Autodesk Inventor part; units mm, degrees
ref_plane "YZ Plane" through (0, 0, 0) normal (1, 0, 0) x (0, 1, 0)
ref_plane "XZ Plane" through (0, 0, 0) normal (0, 1, 0) x (-1, 0, 0)
ref_plane "XY Plane" through (0, 0, 0) normal (0, 0, 1) x (1, 0, 0)
sketch "Sketch1" plane through (0, 0, 0) normal (0, 1, 0) x (-1, 0, 0)
  circle A0 centre (0, 0) radius 6.35
  circle A1 centre (0, 0) radius 3.175
  line L0 (0, 0) -> (-25.4, 0)
  line L1 (0, 0) -> (12.7, -21.997)
  line L2 (0, 0) -> (12.7, 21.997)
  line L3 (12.0126, 22.3939) -> (13.3874, 21.6002)
  line L4 (13.3874, 21.6002) -> (-0.6874, 0.3969) construction
  line L5 (0.6874, -0.3969) -> (12.0126, 22.3939) construction
  line L6 (0, -0.7937) -> (0, 0)
  line L7 (0, 0.7937) -> (-25.4, -0.7937) construction
  line L8 (-25.4, 0.7937) -> (0, -0.7937) construction
  line L9 (0.6874, 0.3969) -> (12.0126, -22.3939) construction
  line L10 (13.3874, -21.6002) -> (-0.6874, -0.3969) construction
  line L11 (-25.4, -0.7937) -> (-3.0742, -0.7937)
  line L12 (-3.0742, 0.7937) -> (-25.4, 0.7937)
  line L13 (0.8497, 3.0592) -> (12.0126, 22.3939)
  line L14 (13.3874, 21.6002) -> (2.2245, 2.2654)
  line L15 (2.2245, -2.2654) -> (13.3874, -21.6002)
  line L16 (12.0126, -22.3939) -> (0.8497, -3.0592)
  line L17 (-25.4, 0) -> (-50.8, 0)
  line L18 (12.7, -21.997) -> (25.4, -43.9941)
  line L19 (12.7, 21.997) -> (25.4, 43.9941)
  line L20 (26.0874, 43.5972) -> (13.3874, 21.6002)
  line L21 (13.3874, 21.6002) -> (12.0126, 22.3939)
  line L22 (12.0126, 22.3939) -> (24.7126, 44.391)
  line L23 (24.7126, 44.391) -> (26.0874, 43.5972)
  line L24 (26.0874, 43.5972) -> (12.0126, 22.3939) construction
  line L25 (13.3874, 21.6002) -> (24.7126, 44.391) construction
  line L26 (26.0627, -43.5544) -> (12.0373, -22.4367) construction
  line L27 (13.4121, -21.643) -> (24.6879, -44.3482) construction
  line L28 (-50.8, 0.7937) -> (-25.4, 0.7937)
  line L29 (-25.4, -0.7937) -> (-50.8, -0.7937)
  line L30 (-50.8, -0.7937) -> (-50.8, 0.7937)
  line L31 (-50.8, 0.7937) -> (-25.4, -0.7937) construction
  line L32 (-25.4, 0.7937) -> (-50.8, -0.7937) construction
  line L33 (24.7126, -44.391) -> (12.0126, -22.3939)
  line L34 (13.3874, -21.6002) -> (26.0874, -43.5972)
  line L35 (26.0874, -43.5972) -> (24.7126, -44.391)
  line L36 (24.7126, -44.391) -> (13.3874, -21.6002) construction
  line L37 (12.0126, -22.3939) -> (26.0874, -43.5972) construction
  point P0 (6.35, 10.9985)
  point P1 (-12.7, 0)
  point P2 (6.35, -10.9985)
  point P3 (3.8375, -5.0593)
  point P4 (3.175, -5.4993)
  point P5 (-6.3002, -0.7937)
  point P6 (2.4627, -5.853)
  point P7 (3.8375, 5.0593)
  point P8 (2.4627, 5.853)
  point P9 (-6.3002, 0.7938)
  point P10 (19.05, 32.9956)
  point P11 (19.05, -32.9956)
  point P12 (-38.1, 0)
extrude "Extrusion1" add sketch "Sketch1" along normal blind 12.7 contours A0 L15 A1 L14 | L14 A1 L2 A0 | A0 L2 L3 L14 | L15 L34 L35 L18 L1 A0 | A0 L1 A1 L15 | L2 A1 L13 A0 | A0 L13 L3 L2 | L3 L19 L23 L20 | L1 L18 L35 L33 L16 A0 | A0 L16 A1 L1 | L13 A1 L12 A0 | L3 L22 L23 L19 | A0 L11 A1 L16 | L12 A1 L0 A0 | A0 L0 L17 L30 L28 L12 | L11 L29 L30 L17 L0 A0 | A0 L0 A1 L11
properties part number "brush_tpu_test_print"
Source: CAD feature listing. Evaluate the final solid. Frame: model axes, mm. A direction names the side the tool comes from. Round coordinates to 2 decimals unless told otherwise and drop trailing zeros. Loops run counter-clockwise (first coordinate to the right, second up) from the corner with the lowest first, then second, coordinate; pieces in that order, holes last. Notation, with made-up numbers: M 33,-18 L 60,-18 A28 cw 60,10 Z; hole C 80.5,48.5 d7. An arc over 180 degrees is marked long. Use a Markdown table: item, result. Add a question column.
1. Section query D-D on z = -38. Return the cut outline in (x, y), then the cut area to 3 significant figures.
2. Section query A-A on x = 0. Return the cut outline in (y, z) (3 decimals).
3. Section query B-B on y = 4.5. Return the cut outline in (x, z) (3 decimals), then the cut area to 3 significant figures.
4. Line query: line 1 (X direction, y = 8.25, z = 0) (3 decimals); line 2 (Z direction, x = 0, y = 8.25) (3 decimals); line 3 (Z direction, x = 1.5, y = 12.25). Output: solid intervals per line, ascending.
5. Contact query for flat-ended pins moving along their axis: P1, Ø6.5, axis at x = 17.5, y = 7.5, coming from the -Z side; P2, Ø6.5, axis at x = 29, y = 5.5, coming from the +Z side; P3, Ø1.5, axis at y = 1.5, z = 21, coming from the +X side. Output: stop coordinate, or through.
6. Mould query, pull axis X, two halves, no side actions, for faces 4 (the flat face through (4, 12.7, 0)), 5 (the cylindrical face through (3.246, 6.261, 5.458)), 6 (the cylindrical face through (-6.35, 6.26, 0.08)). Classes: pulls with the +X half, pulls with the -X half, needs draft (parallel to the pull), parting line crosses it, or undercut.
7. Section query C-C on x = 31. Return the cut outline in (y, z).
8. Reachability of faces 1 (the flat face through (28, 6, 0.794)), 2 (the cylindrical face through (0.69, 6.26, 3.1)), 3 (the flat face through (29, 6, -0.794)) from +Z, -Z, +X, -X, +Y, -Y: full face, straight path, thin tool, end or side. Return the list, or none.
Reported:
| question | item | result |
|---|---|---|
| 1 | outline | M -22.86,0 L -21.02,0 L -21.02,12.7 L -22.86,12.7 Z |
| 1 | area | 23.3 mm² |
| 2 | outline | M 0,-6.35 L 12.7,-6.35 L 12.7,-3.175 L 0,-3.175 Z; M 0,3.175 L 12.7,3.175 L 12.7,6.35 L 0,6.35 Z |
| 3 | outline | M -26.087,-43.597 L -24.713,-44.391 L -12.013,-22.394 L -2.463,-5.853 A6.35 ccw 6.3,-0.794 L 50.8,-0.794 L 50.8,0.794 L 6.3,0.794 A6.35 ccw -2.463,5.853 L -12.013,22.394 L -24.713,44.391 L -26.087,43.597 L -13.387,21.6 L -3.838,5.059 A6.35 ccw -3.838,-5.059 L -13.387,-21.6 Z; hole C 0,0 d6.35 |
| 3 | area | 307 mm² |
| 4 | line 1 | x = -6.35 to -3.175, 3.175 to 50.8 |
| 4 | line 2 | z = -6.35 to -3.175, 3.175 to 6.35 |
| 4 | line 3 | z = -6.17 to -2.8, 2.8 to 6.17 |
| 5 | P1 | stops at z = -0.79 |
| 5 | P2 | stops at z = 0.79 |
| 5 | P3 | stops at x = -10.77 |
| 6 | face 4 | needs draft |
| 6 | face 5 | undercut |
| 6 | face 6 | pulls with the -X half |
| 7 | outline | M 0,-0.79 L 12.7,-0.79 L 12.7,0.79 L 0,0.79 Z |
| 8 | face 1 | +Z, +X, +Y, -Y |
| 8 | face 2 | +Y, -Y |
| 8 | face 3 | -Z, +X, +Y, -Y |
